Drawing for the job (mm, zero at the part's lowest x, y, z). Round coordinates to 2 decimals unless told otherwise and drop trailing zeros. Loops run counter-clockwise (first coordinate to the right, second up) from the corner with the lowest first, then second, coordinate; pieces in that order, holes last. Notation, with made-up numbers: M -17,54 L 36,54 A8 cw 36,64 Z; hole C -31.5,31 d4. An arc over 180 degrees is marked long. Answer in a Markdown table with one row per item.
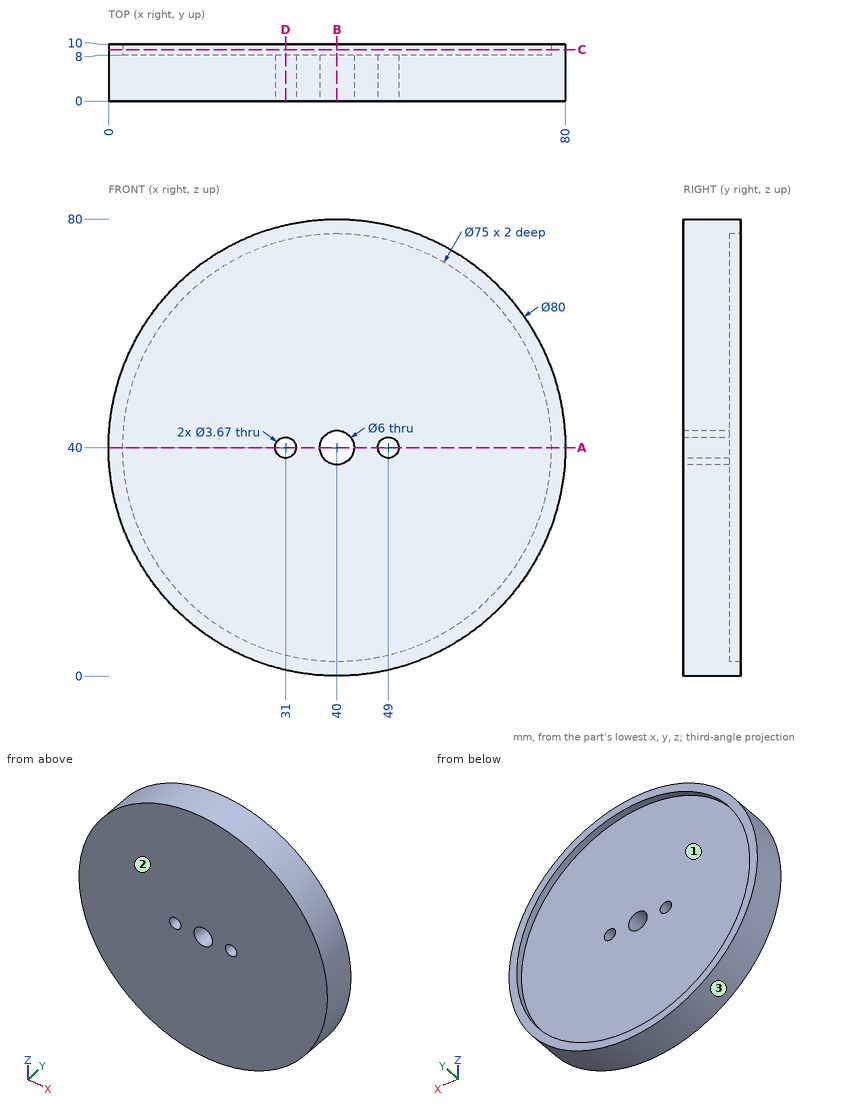
1. Saw through at A-A (z = 40). Write the cut outline in (x, y) (3 decimals), and give its area (3 significant figures).
Verdict:
| item | result |
|---|---|
| outline | M 0,0 L 29.165,0 L 29.165,8 L 2.5,8 L 2.5,10 L 0,10 Z; M 32.835,0 L 37,0 L 37,8 L 32.835,8 Z; M 43,0 L 47.165,0 L 47.165,8 L 43,8 Z; M 50.835,0 L 80,0 L 80,10 L 77.5,10 L 77.5,8 L 50.835,8 Z |
| area | 543 mm² |
2. Mould opens along Z. For the marked faces 1, 2 and 3 say: +Z half, -Z half, draft (parallel to the pull), parting line (faces both ways), or undercut.
Verdict:
| item | result |
|---|---|
| face 1 | undercut |
| face 2 | draft |
| face 3 | parting line |
3. Saw through at B-B (x = 40). Write the cut outline in (y, z).
Verdict:
| item | result |
|---|---|
| outline | M 0,0 L 10,0 L 10,2.5 L 8,2.5 L 8,37 L 0,37 Z; M 0,43 L 8,43 L 8,77.5 L 10,77.5 L 10,80 L 0,80 Z |
4. Saw through at C-C (y = 9). Write the cut outline in (x, z), and give its area (3 significant figures).
Verdict:
| item | result |
|---|---|
| outline | C 40,40 d80; hole C 40,40 d75 |
| area | 609 mm² |
5. Pin check, flat tips, straight feed: pin 1 (4 mm diameter, centred on x = 67, y = 7.5, fed in from -Z) (3 decimals); pin 2 (5 mm diameter, centred on y = 4, z = 19, fed in from +X); pin 3 (8 mm diameter, centred on x = 40, z = 40, fed in from +Y). Stop position of each tip, or through.
Verdict:
| item | result |
|---|---|
| pin 1 | stops at z = 8.775 |
| pin 2 | stops at x = 75.46 |
| pin 3 | stops at y = 8 |
6. Wall check: probe 1 along X at (y, z) = (5.25, 40) (3 decimals); probe 2 along X at (y, z) = (8.75, 40); probe 3 along Y at (x, z) = (42.5, 42). Give the ranges that are in metal, low to high.
Verdict:
| item | result |
|---|---|
| probe 1 | x = 0 to 29.165, 32.835 to 37, 43 to 47.165, 50.835 to 80 |
| probe 2 | x = 0 to 2.5, 77.5 to 80 |
| probe 3 | y = 0 to 8 |
7. Saw through at D-D (x = 31). Write the cut outline in (y, z) (3 decimals), and give its area (3 significant figures).
Verdict:
| item | result |
|---|---|
| outline | M 0,1.026 L 10,1.026 L 10,3.596 L 8,3.596 L 8,38.165 L 0,38.165 Z; M 0,41.835 L 8,41.835 L 8,76.404 L 10,76.404 L 10,78.974 L 0,78.974 Z |
| area | 605 mm² |
